from build123d import *

# Parameters (mm, degrees)
EXTRUDE_1_DEPTH             = 40.5
SKETCH_2_W                  = 38.5
SKETCH_2_H                  = 19.5
CUT_EXTRUDE_1_DEPTH         = 60.752092014
CUT_EXTRUDE_2_DEPTH         = 2
HOLE_WIZARD_3_5_3_5_1_D     = 3.5
HOLE_WIZARD_3_5_3_5_1_DEPTH = 2
HOLE_WIZARD_3_2_3_2_1_D     = 3.2
HOLE_WIZARD_3_2_3_2_1_DEPTH = 40.5
FILLET_1_R                  = 1.5
FILLET_2_R                  = 3
FILLET_3_R                  = 3.5
SKETCH_12_R                 = 1.6
CUT_EXTRUDE_3_DEPTH         = 38.5


with BuildPart() as part:
    # 草图1 → 凸台-拉伸1 (new body)
    with BuildSketch(Plane.XY.offset(20.25)):
        with BuildLine():
            Line((20, -2), (20, 19.5))
            ThreePointArc((20, 19.5), (0, 39.5), (-20, 19.5))
            Line((-20, 19.5), (-20, -2))
            Line((-20, -2), (20, -2))
        make_face()
    extrude(amount=-EXTRUDE_1_DEPTH)

    # 草图2 → 切除-拉伸1 (cut, through all)
    with BuildSketch(Plane(origin=(20, 0, 0), x_dir=(0, 0, -1), z_dir=(1, 0, 0))):
        with Locations((1, 9.75)):
            Rectangle(SKETCH_2_W, SKETCH_2_H)
    extrude(amount=-CUT_EXTRUDE_1_DEPTH, mode=Mode.SUBTRACT)

    # 草图3 → 切除-拉伸2 (cut)
    with BuildSketch(Plane.XY.offset(20.25)):
        with BuildLine():
            Line((-6.5, 26.5), (-6.5, 12.5))
            ThreePointArc((-6.5, 12.5), (0, 6), (6.5, 12.5))
            Line((6.5, 12.5), (6.5, 26.5))
            ThreePointArc((6.5, 26.5), (0, 33), (-6.5, 26.5))
        make_face()
    extrude(amount=-CUT_EXTRUDE_2_DEPTH, mode=Mode.SUBTRACT)

    # Ø3.5 (3.5) 直径孔1
    with Locations(Plane(origin=(0, -2, 0), x_dir=(-1, 0, 0), z_dir=(0, -1, 0))):
        with Locations((15, -11.25), (15, 12.75), (-15, 12.75), (-15, -11.25)):
            Hole(HOLE_WIZARD_3_5_3_5_1_D / 2, depth=HOLE_WIZARD_3_5_3_5_1_DEPTH)

    # Ø3.2 (3.2) 直径孔1
    with Locations(Plane.XY.offset(20.25)):
        with Locations((-7.75, 32.923393759), (-7.75, 6.076606241), (15.5, 19.5), (7.75, 6.076606241), (-15.5, 19.5), (7.75, 32.923393759)):
            Hole(HOLE_WIZARD_3_2_3_2_1_D / 2, depth=HOLE_WIZARD_3_2_3_2_1_DEPTH)

    # 圆角1
    fillet_1_edges = [part.edges().sort_by_distance(p)[0] for p in [
        (0, 0, 18.25),
    ]]
    fillet(fillet_1_edges, radius=FILLET_1_R)

    # 圆角2
    fillet_2_edges = [part.edges().sort_by_distance(p)[0] for p in [
        (-20, -1, -20.25),
        (20, -1, -20.25),
    ]]
    fillet(fillet_2_edges, radius=FILLET_2_R)

    # 圆角3
    fillet_3_edges = [part.edges().sort_by_distance(p)[0] for p in [
        (0, -2, 20.25),
    ]]
    fillet(fillet_3_edges, radius=FILLET_3_R)

    # 草图12 → 切除-拉伸3 (cut)
    with BuildSketch(Plane(origin=(0, 0, -20.25), x_dir=(-1, 0, 0), z_dir=(0, 0, -1))):
        with BuildLine():
            Line((-20, 19.5), (-17.1, 19.5))
            ThreePointArc((-17.1, 19.5), (-15.5, 21.1), (-13.9, 19.5))
            Line((-13.9, 19.5), (13.9, 19.5))
            ThreePointArc((13.9, 19.5), (15.5, 21.1), (17.1, 19.5))
            Line((17.1, 19.5), (20, 19.5))
            ThreePointArc((20, 19.5), (0, 39.5), (-20, 19.5))
        make_face()
        with Locations(Location((-7.75, 32.923393759, 0), (0, 0, 180))):
            Circle(SKETCH_12_R, mode=Mode.SUBTRACT)
        with Locations(Location((7.75, 32.923393759, 0), (0, 0, 180))):
            Circle(SKETCH_12_R, mode=Mode.SUBTRACT)
    extrude(amount=-CUT_EXTRUDE_3_DEPTH, mode=Mode.SUBTRACT)


solid = part.part
Source: CAD feature listing. Evaluate the final solid. Frame: model axes, mm. A direction names the side the tool comes from. Give positions to 0.01 mm unless a question says otherwise; leave off trailing zeros. Write each loop counter-clockwise with the first axis right and the second up, starting at its lowest first coordinate (ties: lowest second). Pieces come first, ordered by that corner, then holes. Notation, with made-up numbers: M 29.25,-15 L 43.25,-15 A7 ccw 43.25,-5 Z; hole C 39.25,29.5 d5. An arc over 180 degrees is marked long. Return JSON: item names as keys, results as strings. Group by question number.
1) Pull-direction query (X, two-part tool) for faces 4 (the face through (-19.1, -1.01, -19.39)), 5 (the face through (-14.059, -0.986, -14.226)), 6 (the face through (-0.28, 0.45, 17.82)), 7 (the face through (15.941, -0.986, 9.774)); classes: pulls with the +X half, pulls with the -X half, needs draft (parallel to the pull), parting line crosses it, or undercut.
2) Set-up query: faces 1 (the face through (0, 0, -1)), 2 (the face through (0, 6, 19)), 3 (the face through (0.44, 39.495, 19.264)). Return all of +Z, -Z, +X, -X, +Y, -Y with unobstructed straight access to the full face (end or side cutting, diameter ignored); none if empty.
3) Cut plane B-B, the plane x = 0. Output: boundary loops of the cut face in (y, z).
4) Cut plane C-C, the plane y = 11.5. Output: boundary loops of the cut face in (x, z).
5) Pin query (flat end, axial travel): P1, Ø4, axis at x = 7.75, y = 6.08, coming from the -Z side; P2, Ø2.5, axis at x = -15.5, y = 19.5, coming from the -Z side; P3, Ø18.5, axis at x = -2, z = 3, coming from the +Y side; P4, Ø1, axis at y = 21, z = 19.5, coming from the -X side (3 decimals). Return the tip coordinate at first contact, or that it passes through.
6) Material intervals for line 1 along X through (y, z) = (-0.6, -12.75); line 2 along X through (y, z) = (19.5, 19.3); line 3 along Z through (x, y) = (15, -1.5), sorted ascending. Write a range as [from, to].
7) Cut plane A-A, the plane z = 11.25. Output: boundary loops of the cut face in (x, y).
8) Cut plane D-D, the plane x = 7.75. Output: boundary loops of the cut face in (y, z).
Recorded:
{
 "1": {"face 4": "pulls with the -X half", "face 5": "undercut", "face 6": "needs draft", "face 7": "undercut"},
 "2": {"face 1": "-Z, +X, -X, +Y", "face 2": "+Z, -Z", "face 3": "+Z, -Z, +Y"},
 "3": {"outline": "M -2,-20.25 L 0,-20.25 L 0,16.75 A1.5 cw 1.5,18.25 L 6,18.25 L 6,20.25 L 1.5,20.25 A3.5 ccw -2,16.75 Z; M 33,18.25 L 39.5,18.25 L 39.5,20.25 L 33,20.25 Z"},
 "4": {"outline": "M -20,18.25 L -6.42,18.25 L -6.42,20.25 L -20,20.25 Z; M 6.42,18.25 L 20,18.25 L 20,20.25 L 6.42,20.25 Z"},
 "5": {"P1": "stops at z = 18.25", "P2": "passes through", "P3": "stops at y = 0", "P4": "stops at x = -19.975"},
 "6": {"line 1": "x = [-20, -16.75], [-13.25, 13.25], [16.75, 20]", "line 2": "x = [-20, -17.1], [-13.9, -6.5], [6.5, 13.9], [17.1, 20]", "line 3": "z = [-20.25, -14.5], [-11, 9.5], [13, 18.55]"},
 "7": {"outline": "M -20,-2 L -16.75,-2 L -16.75,0 L -20,0 Z; M -13.25,-2 L 13.25,-2 L 13.25,0 L -13.25,0 Z; M 16.75,-2 L 20,-2 L 20,0 L 16.75,0 Z"},
 "8": {"outline": "M -2,-20.25 L 0,-20.25 L 0,16.75 A1.5 cw 1.5,18.25 L 4.48,18.25 L 4.48,20.25 L 1.5,20.25 A3.5 ccw -2,16.75 Z; M 7.68,18.25 L 31.32,18.25 L 31.32,20.25 L 7.68,20.25 Z; M 34.52,18.25 L 37.94,18.25 L 37.94,20.25 L 34.52,20.25 Z"}
}
